from build123d import *

# Parameters (mm, degrees)
SKETCH1_R           = 1.5
BOSS_EXTRUDE1_DEPTH = 15
SKETCH2_W           = 5
SKETCH2_H           = 4.697023624
CUT_EXTRUDE1_DEPTH  = 30
SKETCH3_R           = 1
CUT_EXTRUDE2_DEPTH  = 30


with BuildPart() as part:
    # Sketch1 → Boss-Extrude1 (new body)
    with BuildSketch(Plane.XY):
        Circle(SKETCH1_R)
    extrude(amount=BOSS_EXTRUDE1_DEPTH)

    # Sketch2 → Cut-Extrude1 (cut)
    with BuildSketch(Plane(origin=(0, 0, 0), x_dir=(0, 0, -1), z_dir=(1, 0, 0))):
        with Locations((-2.5, -0.042086347)):
            Rectangle(SKETCH2_W, SKETCH2_H)
    extrude(amount=-CUT_EXTRUDE1_DEPTH, mode=Mode.SUBTRACT)

    # Sketch3 → Cut-Extrude2 (cut)
    with BuildSketch(Plane.ZY):
        with Locations((2.282543491, 0)):
            Circle(SKETCH3_R)
    extrude(amount=-CUT_EXTRUDE2_DEPTH, mode=Mode.SUBTRACT)


solid = part.part
Verification items for the finished model (mm, model axes). A direction names the side the tool comes from. Coordinates: 2 decimals unless noted, no trailing zeros. Write each loop counter-clockwise with the first axis right and the second up, starting at its lowest first coordinate (ties: lowest second). Pieces come first, ordered by that corner, then holes. Notation, with made-up numbers: M 20.5,73 L 79.5,73 A4 cw 79.5,79 Z; hole C 5.5,-7.5 d10. An arc over 180 degrees is marked long. One line per question, with ' | ' between items.
1) Access from +Z, -Z, +X, -X, +Y, -Y to the whole of each face (thin tool, end or side, straight path). Record for faces 1 (the face through (0, 0, 15)), 2 (the face through (0, 1, 3)).
Solutions:
face 1: +Z, +X, -X, +Y, -Y | face 2: -Z, -X, +Y, -Y
2) Sectioned sample at A-A on y = 0. Record the cut outline in (x, z), then the cut area to 3 significant figures.
Solutions:
outline: M -1.5,5 L 0,5 L 0,3.28 L 1.5,3.28 L 1.5,15 L -1.5,15 Z; M 0,0 L 1.5,0 L 1.5,1.28 L 0,1.28 Z | area: 34.5 mm^2
3) Material ranges on L1, parallel to Z at x = 0.8, y = 0; L2, parallel to X at y = 0.1, z = 14.5; L3, parallel to Z at x = -1.2, y = -0.55, recorded low to high.
Solutions:
L1: 0 to 1.28, 3.28 to 15 | L2: -1.5 to 1.5 | L3: 5 to 15
4) Depth check by flat-ended pin: pin 1 Ø1.5 at (y, z) = (-0.5, 1.5) entering from -X; pin 2 Ø1 at (x, y) = (0.5, 1) entering from -Z; pin 3 Ø1 at (x, z) = (-1, 9) entering from +Y; pin 4 Ø1.5 at (y, z) = (-1, 6.5) entering from -X. Enter the tip coordinate at first touch or a pass-through.
Solutions:
pin 1: x = 0 | pin 2: z = 0 | pin 3: y = 1.41 | pin 4: x = -1.48
5) Sectioned sample at D-D on x = 0.5. Record the cut outline in (y, z), then the cut area to 3 significant figures.
Solutions:
outline: M -1.41,0 L 1.41,0 L 1.41,15 L -1.41,15 Z; hole C 0,2.28 d2 | area: 39.3 mm^2
6) Sectioned sample at B-B on x = 1.25. Record the cut outline in (y, z).
Solutions:
outline: M -0.83,0 L 0.83,0 L 0.83,1.72 A1 cw -0.83,1.72 Z; M -0.83,2.84 A1 cw 0.83,2.84 L 0.83,15 L -0.83,15 Z
7) Sectioned sample at C-C on z = 3. Record the cut outline in (x, y), then the cut area to 3 significant figures.
Solutions:
outline: M 0,-1.5 A1.5 ccw 1.33,-0.7 L 0,-0.7 Z; M 0,0.7 L 1.33,0.7 A1.5 ccw 0,1.5 Z | area: 1.52 mm^2
8) Release check for a two-part mould opening along Y. For faces 3 (the face through (1.43, 0.45, 9.06)), 4 (the face through (0.74, 0.843, 2.82)), 5 (the face through (1, 0, 0)) record: +Y half, -Y half, draft (parallel to the pull), parting line (faces both ways), or undercut.
Solutions:
face 3: parting line | face 4: undercut | face 5: draft
